Work out the finished part from the listing and answer in its coordinate system (mm). Give positions to 0.01 mm unless a question says otherwise; leave off trailing zeros. Write each loop counter-clockwise with the first axis right and the second up, starting at its lowest first coordinate (ties: lowest second). Pieces come first, ordered by that corner, then holes. Notation, with made-up numbers: (-35.75, 16) - (13.25, 16) arc R12 cw to (13.25, 31) - close; hole circle Ø9 at (-16.75, 35.5). An arc over 180 degrees is marked (long way). Write item = value, one per line.
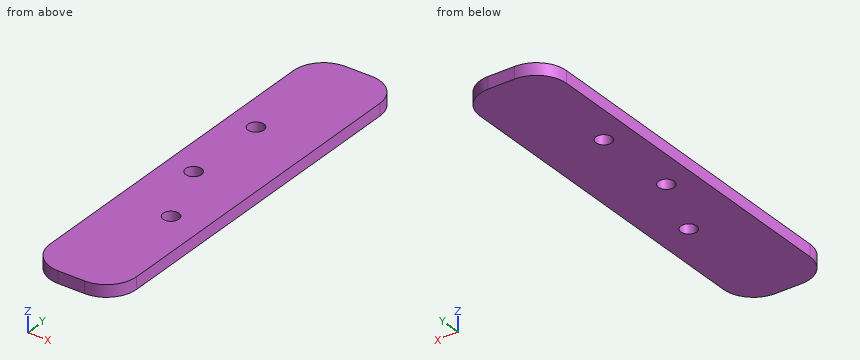
from build123d import *

# Parameters (mm, degrees)
SKETCH1_W            = 28.802861634
SKETCH1_H            = 131.078546172
BOSS_EXTRUDE1_DEPTH  = 4
M5_CLEARANCE_HOLE1_D = 5.3
FILLET1_R            = 10
M5_CLEARANCE_HOLE2_D = 5.3


with BuildPart() as part:
    # Sketch1 → Boss-Extrude1 (new body)
    with BuildSketch(Plane.XY):
        with Locations((-48.87450938, -319.394379884)):
            Rectangle(SKETCH1_W, SKETCH1_H)
    extrude(amount=BOSS_EXTRUDE1_DEPTH)

    # M5 Clearance Hole1 (through all)
    with Locations(Plane.XY.offset(4)):
        with Locations((-54.16270611, -321.915681156), (-54.16270611, -293.415681156)):
            Hole(M5_CLEARANCE_HOLE1_D / 2)

    # Fillet1
    fillet1_edges = [part.edges().sort_by_distance(p)[0] for p in [
        (-63.275940197, -253.855106798, 2),
        (-34.473078563, -253.855106798, 2),
        (-34.473078563, -384.93365297, 2),
        (-63.275940197, -384.93365297, 2),
    ]]
    fillet(fillet1_edges, radius=FILLET1_R)

    # M5 Clearance Hole2 (through all)
    with Locations(Plane(origin=(0, 0, 0), x_dir=(-1, 0, 0), z_dir=(0, 0, -1))):
        with Locations((45.426427008, -344.165502047)):
            Hole(M5_CLEARANCE_HOLE2_D / 2)


solid = part.part
1. Find section A-A, the plane z = 2.15. Give the vertices of the cut face in (x, y).
Solution:
outline = (-63.28, -374.93) arc R10 ccw to (-53.28, -384.93) - (-44.47, -384.93) arc R10 ccw to (-34.47, -374.93) - (-34.47, -263.86) arc R10 ccw to (-44.47, -253.86) - (-53.28, -253.86) arc R10 ccw to (-63.28, -263.86) - close; hole circle Ø5.3 at (-54.16, -321.92); hole circle Ø5.3 at (-54.16, -293.42); hole circle Ø5.3 at (-45.43, -344.17)
2. Find section B-B, the plane x = -58.5. Give the vertices of the cut face in (y, z).
Solution:
outline = (-383.46, 0) - (-255.33, 0) - (-255.33, 4) - (-383.46, 4) - close
3. Given pin 1 (1.5 mm diameter, centred on x = -42, z = 2, fed in from +Y), flat-ended and moving along its own axis, determine where the tip first touches the part or whether it passes through.
Solution:
pin_1 = -254
4. Straight lines are drawn through the part: line 1 (Y direction, x = -54.25, z = 1); line 2 (Y direction, x = -52.25, z = 3.15); line 3 (Y direction, x = -45.25, z = 2.1). For each, find the intervals that lie inside material, in ascending order.
Solution:
line_1 = -384.89 to -324.56, -319.27 to -296.06, -290.77 to -253.9
line_2 = -384.93 to -323.75, -320.08 to -295.25, -291.58 to -253.86
line_3 = -384.93 to -346.81, -341.52 to -253.86
